Build history of the part. All positions in model axes, mm. A direction names the side the tool comes from. Round coordinates to 2 decimals unless told otherwise and drop trailing zeros. Order: outer loops, then holes, each group sorted by start corner. A loop starts at its lowest first (then second) coordinate and runs counter-clockwise, first axis right, second up. Notation, with made-up numbers: (85.5, 41.5) -> (126.5, 41.5) arc R18 ccw to (126.5, 63.5) -> close; hole circle Ø10 at (42, 71.5). An arc over 180 degrees is marked (long way). Answer as a JSON object with one key per item and string values.
from build123d import *

# Parameters (mm, degrees)
SKETCH1_W           = 88.9
SKETCH1_H           = 88.9
SKETCH1_R           = 3.175
BOSS_EXTRUDE1_DEPTH = 9.525
SKETCH2_W           = 88.9
SKETCH2_H           = 88.9
BOSS_EXTRUDE2_DEPTH = 3.175
FILLET1_R           = 2.54


with BuildPart() as part:
    # Sketch1 → Boss-Extrude1 (new body)
    with BuildSketch(Plane(origin=(0, 0, 0), x_dir=(1, 0, 0), z_dir=(0, 1, 0))):
        with Locations((44.45, -44.45)):
            Rectangle(SKETCH1_W, SKETCH1_H)
        with Locations((6.35, -82.55)):
            Circle(SKETCH1_R, mode=Mode.SUBTRACT)
        with Locations((82.55, -82.55)):
            Circle(SKETCH1_R, mode=Mode.SUBTRACT)
        Polygon((71.709871939, -76.2), (17.190128061, -76.2), (44.45, -48.940128061), align=None, mode=Mode.SUBTRACT)
        Polygon((12.7, -71.709871939), (12.7, -17.190128061), (39.959871939, -44.45), align=None, mode=Mode.SUBTRACT)
        Polygon((44.45, -39.959871939), (17.190128061, -12.7), (71.709871939, -12.7), align=None, mode=Mode.SUBTRACT)
        with Locations((6.35, -6.35)):
            Circle(SKETCH1_R, mode=Mode.SUBTRACT)
        Polygon((48.940128061, -44.45), (76.2, -17.190128061), (76.2, -71.709871939), align=None, mode=Mode.SUBTRACT)
        with Locations((82.55, -6.35)):
            Circle(SKETCH1_R, mode=Mode.SUBTRACT)
    extrude(amount=BOSS_EXTRUDE1_DEPTH)

    # Sketch2 → Boss-Extrude2 (add)
    with BuildSketch(Plane(origin=(0, 9.525, 0), x_dir=(1, 0, 0), z_dir=(0, 1, 0))):
        with Locations((44.45, -44.45)):
            Rectangle(SKETCH2_W, SKETCH2_H)
        Polygon((44.45, -48.940128061), (71.709871939, -76.2), (17.190128061, -76.2), align=None, mode=Mode.SUBTRACT)
        Polygon((76.2, -17.190128061), (76.2, -71.709871939), (48.940128061, -44.45), align=None, mode=Mode.SUBTRACT)
        Polygon((44.45, -39.959871939), (71.709871939, -12.7), (17.190128061, -12.7), align=None, mode=Mode.SUBTRACT)
        Polygon((12.7, -71.709871939), (39.959871939, -44.45), (12.7, -17.190128061), align=None, mode=Mode.SUBTRACT)
    extrude(amount=BOSS_EXTRUDE2_DEPTH)

    # Fillet1
    fillet1_edges = [part.edges().sort_by_distance(p)[0] for p in [
        (88.9, 6.35, 88.9),
        (0, 6.35, 88.9),
        (0, 6.35, 0),
        (88.9, 6.35, 0),
    ]]
    fillet(fillet1_edges, radius=FILLET1_R)


solid = part.part
1) Probe L1, parallel to X at y = 5, z = 6.35 (3 decimals); L2, parallel to X at y = 9.75, z = 54.5. List the from-to ranges inside material, lowest first. Write a range as from..to.
Checked values:
{"L1": "x = 0..3.175, 9.525..79.375, 85.725..88.9", "L2": "x = 0..12.7, 29.91..38.89, 50.01..58.99, 76.2..88.9"}
2) Flat gauge pin, fed straight in: pin 1 Ø1.9 at (x, z) = (6.5, 8) entering from -Y (3 decimals). Where does the tip first touch, or does it go through?
Checked values:
{"pin 1": "stops at y = 9.525"}
3) Pull direction X, two halves, no side cores. Call faces 4 (the face through (0, 6, 45)), 5 (the face through (83, 9.525, 83)), 6 (the face through (88.9, 6, 45)), 7 (the face through (84.3, 4.7, 79.9)): pulls with the +X half, pulls with the -X half, needs draft (parallel to the pull), parting line crosses it, or undercut.
Checked values:
{"face 4": "pulls with the -X half", "face 5": "undercut", "face 6": "pulls with the +X half", "face 7": "undercut"}
4) Cut at B-B, the plane y = 5.25. Count the separate pieces of the cut face and the enclosed holes in it, plus the area to 3 significant figures.
Checked values:
{"separate pieces": "1", "enclosed holes": "8", "area": "4,800 mm²"}
5) Which spindle directions (+Z, -Z, +X, -X, +Y, -Y) get a long thin tool onto all of the face, cutting with end or side? Do faces 1 (the face through (45, 6, 76.2)), 2 (the face through (83, 9.525, 6)), 3 (the face through (0.724, 6.261, 0.764)). Say none if no direction does.
Checked values:
{"face 1": "+Y, -Y", "face 2": "-Y", "face 3": "-Z, -X, +Y, -Y"}
6) Cut at A-A, the plane z = 82.55. Give the cut face in (x, y) (3 decimals), plus the area to 3 significant figures.
Checked values:
{"outline": "(0, 0) -> (3.175, 0) -> (3.175, 9.525) -> (9.525, 9.525) -> (9.525, 0) -> (79.375, 0) -> (79.375, 9.525) -> (85.725, 9.525) -> (85.725, 0) -> (88.9, 0) -> (88.9, 12.7) -> (0, 12.7) -> close", "area": "1,010 mm²"}
7) Cut at D-D, the plane z = 25.5. Give the cut face in (x, y).
Checked values:
{"outline": "(0, 0) -> (12.7, 0) -> (12.7, 12.7) -> (0, 12.7) -> close; (21.01, 0) -> (29.99, 0) -> (29.99, 12.7) -> (21.01, 12.7) -> close; (58.91, 0) -> (67.89, 0) -> (67.89, 12.7) -> (58.91, 12.7) -> close; (76.2, 0) -> (88.9, 0) -> (88.9, 12.7) -> (76.2, 12.7) -> close"}
8) Cut at C-C, the plane x = 65.5. Give the cut face in (y, z), plus the area to 3 significant figures.
Checked values:
{"outline": "(0, 0) -> (12.7, 0) -> (12.7, 12.7) -> (0, 12.7) -> close; (0, 18.91) -> (12.7, 18.91) -> (12.7, 27.89) -> (0, 27.89) -> close; (0, 61.01) -> (12.7, 61.01) -> (12.7, 69.99) -> (0, 69.99) -> close; (0, 76.2) -> (12.7, 76.2) -> (12.7, 88.9) -> (0, 88.9) -> close", "area": "551 mm²"}
